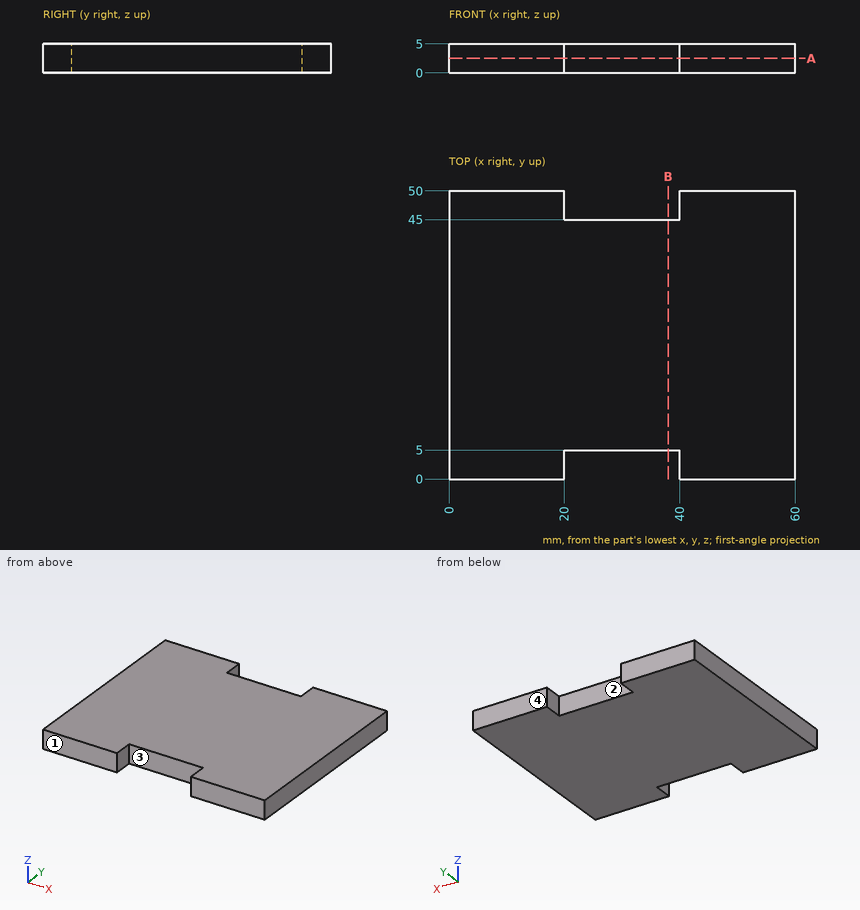
Design review of the part shown in the three views and the two pictorial views. Dimensions are in mm from the part's minimum x, y and z. A direction names the side the tool comes from. Coordinates: 2 decimals unless noted, no trailing zeros. Loops run counter-clockwise (first coordinate to the right, second up) from the corner with the lowest first, then second, coordinate; pieces in that order, holes last.
Q1. The part is to be moulded in two halves that separate along X. For the marked faces 1 and 2, say which applies: +X half, -X half, draft (parallel to the pull), parting line (faces both ways), or undercut.
Reported:
face 1: draft
face 2: undercut
Q2. To check wall thickness, follow line 1 (X direction, y = 47, z = 2.55); line 2 (Y direction, x = 36.5, z = 0.35). State the ranges of each line that lie inside material, in increasing order.
Reported:
line 1: x = 0 to 20, 40 to 60
line 2: y = 5 to 45
Q3. Tool access review of the marked faces 3 and 4: name each direction out of +Z, -Z, +X, -X, +Y, -Y from which nothing blocks a thin tool from reaching the whole face with its end or side.
Reported:
face 3: +Z, -Z, -Y
face 4: +Z, -Z, +X, -X, +Y
Q4. For pin 1 (1 mm diameter, centred on x = 38.5, z = 4.5, fed in from +Y); pin 2 (3 mm diameter, centred on x = 31, z = 3, fed in from -Y), all flat-tipped, find the tip position at first contact; note any pin that passes through.
Reported:
pin 1: stops at y = 45
pin 2: stops at y = 5
Q5. We need section A-A on z = 2.5. State the section outline as (x, y) points.
Reported:
outline: (0, 0) - (20, 0) - (20, 5) - (40, 5) - (40, 0) - (60, 0) - (60, 50) - (40, 50) - (40, 45) - (20, 45) - (20, 50) - (0, 50) - close
Q6. We need section B-B on x = 38. State the section outline as (y, z) points.
Reported:
outline: (5, 0) - (45, 0) - (45, 5) - (5, 5) - close
